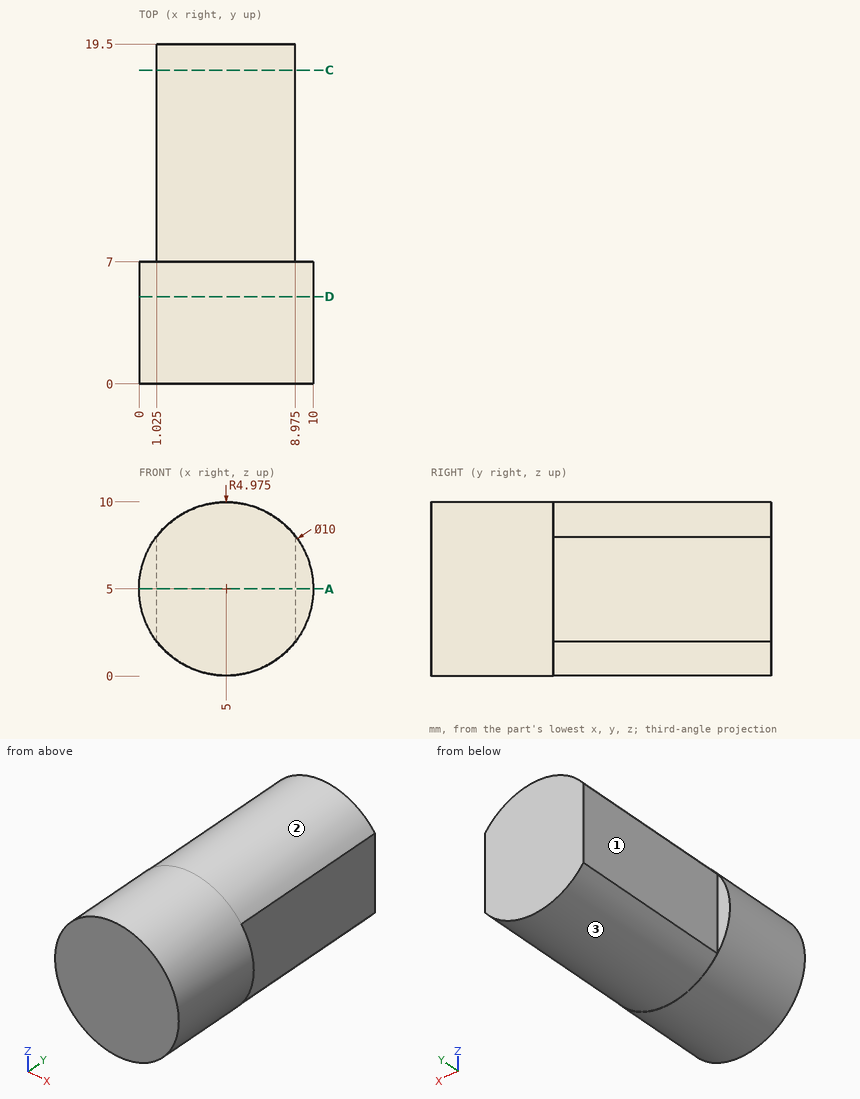
For this review, use the dimensioned drawing (mm, ordinates from the lowest corner) and the shaded views. A direction names the side the tool comes from. Give positions to 0.01 mm unless a question says otherwise; leave off trailing zeros. Write each loop counter-clockwise with the first axis right and the second up, starting at its lowest first coordinate (ties: lowest second). Pieces come first, ordered by that corner, then holes. Notation, with made-up numbers: M 22,9.25 L 48,9.25 A24 cw 48,25.25 Z; hole C 56.25,12 d2. An arc over 180 degrees is marked long. Write item = value, one per line. Start each with the question number.
Q1. We need section C-C (y = 18). State the section outline as (x, z) points (3 decimals), plus the area to 3 significant figures.
Q2. For line 1 (X direction, y = 9, z = 5.5) (3 decimals); line 2 (X direction, y = 6.25, z = 5.5); line 3 (Z direction, x = 2, y = 7.5), list the stretches that pass through material, from the lowest coordinate up.
Q3. We need section D-D (y = 5). State the section outline as (x, z) points, plus the area to 3 significant figures.
Q4. Clearance check with flat-ended pins moving along their axes: pin 1 (4 mm diameter, centred on x = 4, z = 6, fed in from -Y); pin 2 (4 mm diameter, centred on x = 7.5, y = 3, fed in from -Z); pin 3 (1.8 mm diameter, centred on y = 11.5, z = 5, fed in from -X) (3 decimals); pin 4 (2 mm diameter, centred on x = 2.5, y = 11, fed in from -Z). State where each tip first meets the part, or that it passes through.
Q5. We need section A-A (z = 5). State the section outline as (x, y) points (3 decimals).
Q6. Machinability: for the marked faces 1, 2 and 3, which of the approach directions +Z, -Z, +X, -X, +Y, -Y give a long, thin tool a straight path to every point of the face, cutting with its end or side? Answer none if there is none.
Result set:
q1.outline = M 1.025,2.008 A4.975 ccw 8.975,2.008 L 8.975,7.992 A4.975 ccw 1.025,7.992 Z
q1.area = 69.6 mm2
q2.line_1 = 1.025 to 8.975
q2.line_2 = 0.03 to 9.97
q2.line_3 = 1.03 to 8.97
q3.outline = C 5,5 d10
q3.area = 78.5 mm2
q4.pin_1 = 0
q4.pin_2 = 0.03
q4.pin_3 = 1.025
q4.pin_4 = 0.26
q5.outline = M 0,0 L 10,0 L 10,7 L 8.975,7 L 8.975,19.5 L 1.025,19.5 L 1.025,7 L 0,7 Z
q6.face_1 = +Z, -Z, -X, +Y
q6.face_2 = +Z, +Y
q6.face_3 = -Z, +Y
